Read the model definition and answer for the solid it produces. Units are mm, in the model's axes. A direction names the side the tool comes from. Coordinates: 2 decimals unless noted, no trailing zeros. Loops run counter-clockwise (first coordinate to the right, second up) from the corner with the lowest first, then second, coordinate; pieces in that order, holes last. Notation, with made-up numbers: (74.5, 1) -> (127.5, 1) arc R12 cw to (127.5, 10) -> close; hole circle Ø11 at (68.5, 18). An arc over 180 degrees is marked (long way). Answer as a JSON object with one key per item and string values. Group by question number.
1) Section C-C, the plane y = -53 is taken. Give the vertices of the cut face in (x, z), plus the area to 4 significant figures.
2) Section B-B, the plane x = 32 is taken. Give the vertices of the cut face in (y, z).
3) Section A-A, the plane y = -25.5 is taken. Give the vertices of the cut face in (x, z), plus the area to 3 significant figures.
4) Consider probe 1 along X at (y, z) = (-13, -0.65); probe 2 along Z at (x, y) = (-15.5, -48); probe 3 along Z at (x, y) = (33, -64). Determine where each line is inside the solid, lowest interval first. Write a range as [from, to].
5) Which of the six approach directions +Z, -Z, +X, -X, +Y, -Y give full straight-line access (tool end or side, diameter ignored) to faces 1 (the face through (102.75, -10.5, -0.5)), 2 (the face through (-1, -53, -1))?
6) Flat-ended cylindrical pins translate along their axes: P1, Ø1.5, axis at x = 6, y = -58.5, coming from the -Z side; P2, Ø3, axis at x = -98.02, y = 55.99, coming from the -Z side. Find the tip coordinate at first contact, or state that the pin passes through.
from build123d import *

# Parameters (mm, degrees)
SKETCH_2_W                      = 205.5
SKETCH_2_H                      = 121.5
SM_BASE_FLANGE_1_DEPTH          = 1
SM_EDGE_FLANGE_1_DEPTH          = 205.5
FILLET_1_R                      = 3
SKETCH_12_W                     = 156
SKETCH_12_H                     = 88
CUT_EXTRUDE_2_DEPTH             = 10
FILLET_2_R                      = 0.5
HOLE_WIZARD_M31_D               = 3.4
HOLE_WIZARD_M31_DEPTH           = 8.5
HOLE_WIZARD_M31_TIP             = 1.021463052
HOLE_WIZARD_M31_ON_FACE_2_D     = 3.4
HOLE_WIZARD_M31_ON_FACE_2_DEPTH = 8.5
HOLE_WIZARD_M31_ON_FACE_2_TIP   = 1.021463052
HOLE_WIZARD_M31_ON_FACE_3_D     = 3.4
HOLE_WIZARD_M31_ON_FACE_3_DEPTH = 8.5
HOLE_WIZARD_M31_ON_FACE_3_TIP   = 1.021463052
SKETCH_16_R                     = 1
CUT_EXTRUDE_3_DEPTH             = 10
PATTERN_LINEAR_1_COUNT          = 5
PATTERN_LINEAR_1_PITCH          = 10
PATTERN_LINEAR_1_COL_COUNT      = 5
PATTERN_LINEAR_1_COL_PITCH      = 10
SKETCH_17_R                     = 1
CUT_EXTRUDE_4_DEPTH             = 1
PATTERN_LINEAR_2_COUNT          = 6
PATTERN_LINEAR_2_PITCH          = 10
PATTERN_LINEAR_2_COL_COUNT      = 5
PATTERN_LINEAR_2_COL_PITCH      = 10


# Sheet-metal steps are written as plain solids
with BuildPart() as part:
    # Sketch 2 → Базовая кромка1 (new body)
    with BuildSketch(Plane.XY):
        Rectangle(SKETCH_2_W, SKETCH_2_H)
    extrude(amount=-SM_BASE_FLANGE_1_DEPTH)

    # Ребро-кромка1 section (across the edge) → Ребро-кромка1 (add)
    with BuildSketch(Plane(origin=(102.75, -60.889981862, -1), x_dir=(0, 0.1736481776669237, -0.9848077530122092), z_dir=(-1, 0, 0))):
        with BuildLine():
            Line((-1, 0.139981862), (-1, 19.912511336))
            Line((-1, 19.912511336), (0, 19.912511336))
            Line((0, 19.912511336), (0, 0.139981862))
            ThreePointArc((0, 0.139981862), (0.006088483, 0.000532673), (0.024307595, -0.137855223))
            Line((0.024307595, -0.137855223), (-0.960500158, -0.3115034))
            ThreePointArc((-0.960500158, -0.3115034), (-0.990106215, -0.08662307), (-1, 0.139981862))
        make_face()
    extrude(amount=SM_EDGE_FLANGE_1_DEPTH)

    # Скругление1
    fillet_1_edges = [part.edges().sort_by_distance(p)[0] for p in [
        (102.75, -80.586801497, -3.96536743),
        (-102.75, -80.586801497, -3.96536743),
        (-102.75, 60.75, -0.5),
        (102.75, 60.75, -0.5),
    ]]
    fillet(fillet_1_edges, radius=FILLET_1_R)

    # Эскиз12 → Вырез-Вытянуть2 (cut)
    with BuildSketch(Plane.XY):
        Rectangle(SKETCH_12_W, SKETCH_12_H)
    extrude(amount=-CUT_EXTRUDE_2_DEPTH, mode=Mode.SUBTRACT)

    # Скругление2
    fillet_2_edges = [part.edges().sort_by_distance(p)[0] for p in [
        (-78, -44, -0.5),
        (-78, 44, -0.5),
        (78, 44, -0.5),
        (78, -44, -0.5),
    ]]
    fillet(fillet_2_edges, radius=FILLET_2_R)

    # Сверло под метчик  спиральное M31
    with Locations(Plane(origin=(-98.021320344, -75.77058326, -2.608424904), x_dir=(0, 0.984807753012, 0.173648177667), z_dir=(0, -0.173648177667, 0.984807753012))):
        with Locations((0, 0)):
            Hole(HOLE_WIZARD_M31_D / 2, depth=HOLE_WIZARD_M31_DEPTH)
            with Locations((0, 0, -(HOLE_WIZARD_M31_DEPTH + HOLE_WIZARD_M31_TIP / 2))):  # 118° drill point
                Cone(0, HOLE_WIZARD_M31_D / 2, HOLE_WIZARD_M31_TIP, mode=Mode.SUBTRACT)

    # Сверло под метчик  спиральное M31 on face 2
    with Locations(Plane(origin=(98.021320344, -75.77058326, -2.608424904), x_dir=(0, 0.984807790843, 0.17364796312), z_dir=(0, -0.17364796312, 0.984807790843))):
        with Locations((0, 0)):
            Hole(HOLE_WIZARD_M31_ON_FACE_2_D / 2, depth=HOLE_WIZARD_M31_ON_FACE_2_DEPTH)
            with Locations((0, 0, -(HOLE_WIZARD_M31_ON_FACE_2_DEPTH + HOLE_WIZARD_M31_ON_FACE_2_TIP / 2))):  # 118° drill point
                Cone(0, HOLE_WIZARD_M31_ON_FACE_2_D / 2, HOLE_WIZARD_M31_ON_FACE_2_TIP, mode=Mode.SUBTRACT)

    # Сверло под метчик  спиральное M31 on face 3
    with Locations(Plane(origin=(-98.021320344, 55.994949149, 0), x_dir=(1, 0, 0), z_dir=(0, 0, 1))):
        with Locations((0, 0), (196.042640688, 0)):
            Hole(HOLE_WIZARD_M31_ON_FACE_3_D / 2, depth=HOLE_WIZARD_M31_ON_FACE_3_DEPTH)
            with Locations((0, 0, -(HOLE_WIZARD_M31_ON_FACE_3_DEPTH + HOLE_WIZARD_M31_ON_FACE_3_TIP / 2))):  # 118° drill point
                Cone(0, HOLE_WIZARD_M31_ON_FACE_3_D / 2, HOLE_WIZARD_M31_ON_FACE_3_TIP, mode=Mode.SUBTRACT)

    # Эскиз16 → Вырез-Вытянуть3 (cut)
    with BuildSketch(Plane(origin=(0, -1.838695719, 10.427761604), x_dir=(1, 0, 0), z_dir=(0, -0.17364817766692364, 0.9848077530122092))):
        with Locations(Location((-42.75, -70.164820995, 0), (0, 0, 270))):
            Circle(SKETCH_16_R)
        with Locations(Location((-42.75, -65.164820995, 0), (0, 0, 270))):
            Circle(SKETCH_16_R)
        with Locations(Location((-42.75, -75.164820995, 0), (0, 0, 270))):
            Circle(SKETCH_16_R)
    cut_extrude_3 = extrude(amount=-CUT_EXTRUDE_3_DEPTH, mode=Mode.SUBTRACT)

    # Линейный массив1: Вырез-Вытянуть3 ×5
    with Locations(*[(i * PATTERN_LINEAR_1_PITCH, 0, 0) for i in range(1, PATTERN_LINEAR_1_COUNT)]):
        add(cut_extrude_3, mode=Mode.SUBTRACT)

    # Линейный массив1 col: Вырез-Вытянуть3 ×5
    with Locations(*[(-i * PATTERN_LINEAR_1_COL_PITCH, 0, 0) for i in range(1, PATTERN_LINEAR_1_COL_COUNT)]):
        add(cut_extrude_3, mode=Mode.SUBTRACT)

    # Эскиз17 → Вырез-Вытянуть4 (cut)
    with BuildSketch(Plane(origin=(0, -1.838695719, 10.427761604), x_dir=(1, 0, 0), z_dir=(0, -0.17364817766692364, 0.9848077530122092))):
        with Locations(Location((-47.75, -67.664820995, 0), (0, 0, 270))):
            Circle(SKETCH_17_R)
        with Locations(Location((-47.75, -72.664820995, 0), (0, 0, 270))):
            Circle(SKETCH_17_R)
    cut_extrude_4 = extrude(amount=-CUT_EXTRUDE_4_DEPTH, mode=Mode.SUBTRACT)

    # Линейный массив2: Вырез-Вытянуть4 ×6
    with Locations(*[(i * PATTERN_LINEAR_2_PITCH, 0, 0) for i in range(1, PATTERN_LINEAR_2_COUNT)]):
        add(cut_extrude_4, mode=Mode.SUBTRACT)

    # Линейный массив2 col: Вырез-Вытянуть4 ×5
    with Locations(*[(-i * PATTERN_LINEAR_2_COL_PITCH, 0, 0) for i in range(1, PATTERN_LINEAR_2_COL_COUNT)]):
        add(cut_extrude_4, mode=Mode.SUBTRACT)


solid = part.part
Determined:
{
 "1": {"outline": "(-102.75, -1) -> (102.75, -1) -> (102.75, 0) -> (-102.75, 0) -> close", "area": "205.5 mm²"},
 "2": {"outline": "(-80.67, -3.47) -> (-80.5, -4.46) -> (-61.03, -1.02) arc R1.6 cw to (-60.75, -1) -> (-44, -1) -> (-44, 0) -> (-60.75, 0) arc R2.6 ccw to (-61.2, -0.04) -> close; (44, -1) -> (60.75, -1) -> (60.75, 0) -> (44, 0) -> close"},
 "3": {"outline": "(-102.75, -1) -> (-78, -1) -> (-78, 0) -> (-102.75, 0) -> close; (78, -1) -> (102.75, -1) -> (102.75, 0) -> (78, 0) -> close", "area": "49.5 mm²"},
 "4": {"probe 1": "[-102.75, -78], [78, 102.75]", "probe 2": "[-1, 0]", "probe 3": "[-1.55, -0.53]"},
 "5": {"face 1": "+Z, -Z, +X, +Y, -Y", "face 2": "-Z, +X, -X, +Y"},
 "6": {"P1": "z = -1", "P2": "through"}
}
